Can you work these out from the model? Positions are in its coordinate system, mm. A direction names the side the tool comes from. Coordinates: 2 decimals unless noted, no trailing zeros. Order: outer loops, then holes, each group sorted by start corner. A loop starts at its lowest first (then second) coordinate and runs counter-clockwise, first axis right, second up. Notation, with made-up numbers: M -7.5,-16.75 L 45.5,-16.75 A16 ccw 45.5,6.25 Z; hole C -3.5,-17.5 d11. An arc over 180 degrees is marked long. Answer as CSV lines item,"result". Start each with the question number.
1. If we mould it in two halves opening along X, with no side actions, what happens to faces 1 (the face through (63.744, -12.325, 33.067)), 2 (the face through (-84.75, -12.32, 28.19)), 3 (the face through (-18.1, -25, 29.7))? For each: released by +X, released by -X, zero draft, split by the parting line, or undercut.
2. If we section it at B-B (z = 37): List the corners of the cut face in (x, y) for me.
3. I need wall thicknesses on line 1 along Z through (x, y) = (-70, -7.75); line 2 along X through (y, z) = (-3, 33); line 3 along Z through (x, y) = (-80, -3.25). Which ranges of each line are inside material? Lowest first, please. Write a range as from..to.
4. If we section it at A-A (x = 41.5): List the corners of the cut face in (y, z) for me, plus the area to 3 significant figures.
5. On a 3-axis mill with a long thin cutter (end or side, diameter ignored), from which of +Z, -Z, +X, -X, +Y, -Y can I reach the whole of each face in a straight line? I mean faces 4 (the face through (-14, -12, 29.958)), 5 (the face through (-18.1, 0, 29.7)). Say none if no direction works.
6. Will these pins go through, and if not, where does the flat tip stop? pin 1 (1 mm diameter, centred on x = 19, y = -21, fed in from +Z); pin 2 (1 mm diameter, centred on x = -65, y = -13.5, fed in from -Z).
```python
from build123d import *

# Parameters (mm, degrees)
F0_R     = 1.464722
F1_DEPTH = 25


with BuildPart() as f1:
    # F0 (on Front) → F1 (new body)
    with BuildSketch(Plane.XZ):
        with BuildLine():
            Line((56.823755, 29.957542), (-87.65175, 29.957542))
            add(Edge.make_bspline(
                [(-87.65175, 29.957542), (-88.301932, 29.960531), (-88.75546, 29.505347), (-88.781094, 29.047866)],
                knots=[0, 0, 0, 0, 1.450148, 1.450148, 1.450148, 1.450148], degree=3))
            Line((-88.781094, 29.047866), (-88.781094, 27.945455))
            add(Edge.make_bspline(
                [(-88.781094, 27.945455), (-88.775299, 27.514639), (-88.530844, 27.140533), (-87.988705, 27.056743)],
                knots=[0, 0, 0, 0, 1.190668, 1.190668, 1.190668, 1.190668], degree=3))
            Line((-87.988705, 27.056743), (-83.400639, 27.243855))
            ThreePointArc((-83.400639, 27.243855), (-80.673788, 24.526915), (-81.402029, 28.306749))
            ThreePointArc((-81.402029, 28.306749), (-81.605014, 28.318455), (-81.808144, 28.309632))
            Line((-81.808144, 28.309632), (-87.781094, 28.066041))
            Line((-87.781094, 28.066041), (-87.781094, 28.957542))
            Line((-87.781094, 28.957542), (56.823755, 28.957542))
            ThreePointArc((56.823755, 28.957542), (63.800247, 33.172878), (63.313478, 41.309435))
            Line((63.313478, 41.309435), (62.549877, 40.653716))
            ThreePointArc((62.549877, 40.653716), (62.889985, 33.590834), (56.823755, 29.957542))
        make_face()
        with Locations((-81.619306, 26.304817)):
            Circle(F0_R, mode=Mode.SUBTRACT)
    extrude(amount=F1_DEPTH)


solid = f1.part
```
Solved:
1,face 1,"released by +X"
1,face 2,"undercut"
1,face 3,"zero draft"
2,outline,"M 63.7,-25 L 64.7,-25 L 64.7,0 L 63.7,0 Z"
3,line 1,"28.96..29.96"
3,line 2,"62.53..63.71"
3,line 3,"25.11..27.5, 28.96..29.96"
4,outline,"M -25,28.96 L 0,28.96 L 0,29.96 L -25,29.96 Z"
4,area,"25.0 mm²"
5,face 4,"+Z, -X, +Y, -Y"
5,face 5,"+Z, -Z, +X, -X, +Y"
6,pin 1,"z = 29.96"
6,pin 2,"z = 28.96"
